Autodesk Inventor part; units mm, degrees
ref_plane "YZ Plane" through (0, 0, 0) normal (1, 0, 0) x (0, 1, 0)
ref_plane "XZ Plane" through (0, 0, 0) normal (0, 1, 0) x (-1, 0, 0)
ref_plane "XY Plane" through (0, 0, 0) normal (0, 0, 1) x (1, 0, 0)
sketch "Sketch1" plane through (0, 0, 0) normal (0, 1, 0) x (-1, 0, 0)
  arc A0 (0, -490) -> (-342.9286, 350) centre (0, 0) ccw
  line L0 (0, -490) -> (-650, -490)
  line L1 (-650, -490) -> (-650, 350)
  line L2 (-650, 350) -> (-342.9286, 350)
  dimension "d1" = 980
  dimension "d2" = 350
  dimension "d3" = 650
extrude "Extrusion1" add sketch "Sketch1" along normal mid plane 16
sketch "Sketch2" plane through (0, 8, 0) normal (0, 1, 0) x (1, 0, 0)
  arc A0 (0, 490) -> (342.9286, -350) centre (0, 0) ccw
  line L0 (650, -350) -> (650, 490)
  line L1 (650, 490) -> (0, 490)
  line L2 (435, 465) -> (525, 465)
  line L3 (530, 460) -> (530, 445)
  line L4 (525, 440) -> (435, 440)
  line L5 (430, 445) -> (430, 460)
  arc A1 (435, 465) -> (430, 460) centre (435, 460) ccw
  arc A2 (430, 445) -> (435, 440) centre (435, 445) ccw
  arc A3 (525, 440) -> (530, 445) centre (525, 445) ccw
  arc A4 (530, 460) -> (525, 465) centre (525, 460) ccw
  line L6 (0, 0) -> (-346.4823, 346.4823) construction
  line L7 (-289.9138, 353.5534) -> (-353.5534, 289.9138)
  line L8 (-353.5534, 282.8427) -> (-342.9468, 272.2361)
  line L9 (-335.8757, 272.2361) -> (-272.2361, 335.8757)
  line L10 (-272.2361, 342.9468) -> (-282.8427, 353.5534)
  arc A5 (-353.5534, 289.9138) -> (-353.5534, 282.8427) centre (-350.0179, 286.3782) ccw
  arc A6 (-342.9468, 272.2361) -> (-335.8757, 272.2361) centre (-339.4113, 275.7716) ccw
  arc A7 (-272.2361, 335.8757) -> (-272.2361, 342.9468) centre (-275.7716, 339.4113) ccw
  arc A8 (-282.8427, 353.5534) -> (-289.9138, 353.5534) centre (-286.3782, 350.0179) ccw
  point P0 (430, 465)
  point P1 (530, 465)
  point P2 (430, 440)
  dimension "d6" = 100
  dimension "d7" = 25
  dimension "d8" = 25
  dimension "d9" = 120
  dimension "d10" = 5
  dimension "d11" = 45
  dimension "d15" = 25
  dimension "d16" = 100
  dimension "d17" = 430
  dimension "d18" = 90
  dimension "d19" = 5
extrude "Extrusion2" cut sketch "Sketch2" against normal through all
sketch "Sketch3" plane through (0, 8, 0) normal (0, 1, 0) x (1, 0, 0)
  circle A0 centre (610, 470) radius 4
  circle A1 centre (610, -330) radius 4
  circle A2 centre (610, 70) radius 4
  circle A3 centre (610, 470) radius 2.75
  circle A4 centre (610, 70) radius 2.75
  circle A5 centre (610, -330) radius 2.75
  dimension "d22" = 8
extrude "Extrusion3" cut sketch "Sketch3" against normal through all contours A0 | A1 | A2 | A3 | A4 | A5
ref_plane "Work Plane1" through (0, 0, 0) normal (-0.7071, 0, -0.7071) x (-0.7071, 0, 0.7071)
ref_plane "Work Plane2" through (500, 8, 350) normal (1, 0, 0) x (0, 0, -1)
ref_plane "Work Plane3" through (342.9286, 8, 180) normal (0, 0, 1) x (1, 0, 0)
sketch "Sketch5" plane through (0, -8, 0) normal (0, -1, 0) x (1, 0, 0)
  circle A0 centre (610, 330) radius 4
  circle A1 centre (610, -470) radius 4
  circle A2 centre (610, -70) radius 4
  arc A3 (435, -440) -> (430, -445) centre (435, -445) ccw
  line L0 (435, -440) -> (525, -440)
  arc A4 (530, -445) -> (525, -440) centre (525, -445) ccw
  line L1 (530, -445) -> (530, -460)
  arc A5 (525, -465) -> (530, -460) centre (525, -460) ccw
  line L2 (525, -465) -> (435, -465)
  arc A6 (430, -460) -> (435, -465) centre (435, -460) ccw
  line L3 (430, -460) -> (430, -445)
  arc A7 (-335.8757, -272.2361) -> (-342.9468, -272.2361) centre (-339.4113, -275.7716) ccw
  line L4 (-335.8757, -272.2361) -> (-272.2361, -335.8757)
  arc A8 (-272.2361, -342.9468) -> (-272.2361, -335.8757) centre (-275.7716, -339.4113) ccw
  line L5 (-272.2361, -342.9468) -> (-282.8427, -353.5534)
  arc A9 (-289.9138, -353.5534) -> (-282.8427, -353.5534) centre (-286.3782, -350.0179) ccw
  line L6 (-289.9138, -353.5534) -> (-353.5534, -289.9138)
  arc A10 (-353.5534, -282.8427) -> (-353.5534, -289.9138) centre (-350.0179, -286.3782) ccw
  line L7 (-353.5534, -282.8427) -> (-342.9468, -272.2361)
  arc A11 (342.9286, 350) -> (0, -490) centre (0, 0) ccw
  line L8 (0, -490) -> (650, -490)
  line L9 (650, -490) -> (650, 350)
  line L10 (650, 350) -> (342.9286, 350)
  line L11 (0, 0) -> (650, 0) construction
  line L12 (0, 0) -> (0, -490) construction
properties part number "Base_Left" material "MDF Medium Density Fiberboard"
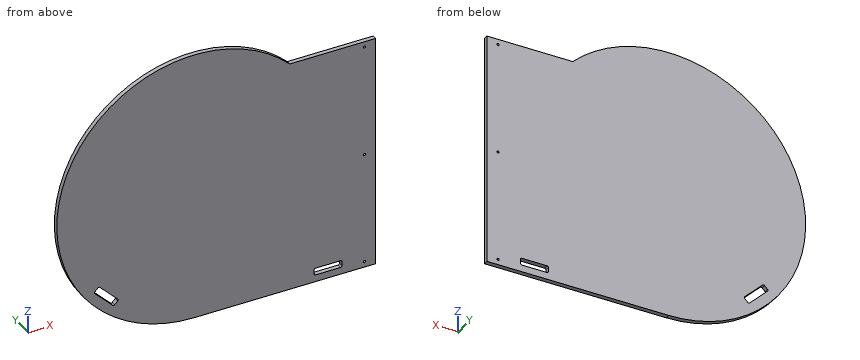
The model under review builds one solid part; all positions refer to its coordinate system, in mm. Coordinates: 2 decimals unless noted, no trailing zeros. Loops run counter-clockwise (first coordinate to the right, second up) from the corner with the lowest first, then second, coordinate; pieces in that order, holes last.
(1) Consider section C-C, the plane z = 389. Give the boundary of the cut face in (x, y), plus the area to 3 significant figures.
Determined:
outline: (-297.96, -8) - (297.96, -8) - (297.96, 8) - (-297.96, 8) - close
area: 9,530 mm2
(2) Consider section A-A, the plane y = 1.5. Give the boundary of the cut face in (x, z), plus the area to 3 significant figures.
Determined:
outline: (0, -490) - (650, -490) - (650, 350) - (342.93, 350) arc R490 ccw (long way) to start; hole (-353.55, -289.91) - (-289.91, -353.55) arc R5 ccw to (-282.84, -353.55) - (-272.24, -342.95) arc R5 ccw to (-272.24, -335.88) - (-335.88, -272.24) arc R5 ccw to (-342.95, -272.24) - (-353.55, -282.84) arc R5 ccw to start; hole (430, -460) arc R5 ccw to (435, -465) - (525, -465) arc R5 ccw to (530, -460) - (530, -445) arc R5 ccw to (525, -440) - (435, -440) arc R5 ccw to (430, -445) - close; hole circle Ø8 at (610, -470); hole circle Ø8 at (610, -70); hole circle Ø8 at (610, 330)
area: 951,000 mm2
(3) Wall thickness on L1, parallel to Z at x = 610, y = -4; L2, parallel to Z at x = 601, y = 0.75; L3, parallel to X at y = -0.75, z = 330: over which ranges is each line inside the solid? List them lowest first.
Determined:
L1: z = -490 to -474, -466 to -74, -66 to 326, 334 to 350
L2: z = -490 to 350
L3: x = -362.22 to 606, 614 to 650
(4) Consider section B-B, the plane x = -182. Give the boundary of the cut face in (y, z), plus the area to 3 significant figures.
Determined:
outline: (-8, -454.95) - (8, -454.95) - (8, 454.95) - (-8, 454.95) - close
area: 14,600 mm2
(5) Insertion check: P1, Ø10.5, axis at x = 610, z = -470, coming from the +Y side; P2, Ø1.5, axis at y = -2, z = -226.5, coming from the -X side; P3, Ø7.5, axis at y = 3.5, z = -450.5, coming from the -X side; P4, Ø6.5, axis at x = 610, z = -70, coming from the +Y side. Each pin has a flat end and moves straight along its axis. Give the tip position at first contact, or say it passes through.
Determined:
P1: stops at y = 8
P2: stops at x = -434.9
P3: stops at x = -201.28
P4: passes through
